```python
from build123d import *

# Parameters (mm, degrees)
PAD_DEPTH    = 10
SKETCH001_R  = 1.5
POCKET_DEPTH = 64.001


with BuildPart() as part:
    # Sketch → Pad (new body)
    with BuildSketch(Plane.XY):
        Polygon((80, 4), (-27.1, 4), (-27.1, -36), (-23.1, -36), (-23.1, 0), (0, 0), (0, -60), align=None)
        Polygon((2, 0), (2, -53.277501), (71.096876, 2), align=None, mode=Mode.SUBTRACT)
    extrude(amount=PAD_DEPTH)

    # Sketch001 (on Face5 of Pad) → Pocket (cut, through all)
    with BuildSketch(Plane(origin=(0, 4, 0), x_dir=(-1, 0, 0), z_dir=(0, 1, 0))):
        with Locations((-60, 5)):
            Circle(SKETCH001_R)
        with Locations((7.1, 5)):
            Circle(SKETCH001_R)
        with Locations((-26.45, 5)):
            Circle(SKETCH001_R)
    extrude(amount=-POCKET_DEPTH, mode=Mode.SUBTRACT)


solid = part.part
```
Part model, mm, in its own coordinate system. A direction names the side the tool comes from. Give positions to 0.01 mm unless a question says otherwise; leave off trailing zeros. Write each loop counter-clockwise with the first axis right and the second up, starting at its lowest first coordinate (ties: lowest second). Pieces come first, ordered by that corner, then holes. Notation, with made-up numbers: (28.25, 52.5) -> (60.25, 52.5) arc R15 ccw to (60.25, 70.5) -> close; hole circle Ø1 at (-15, 35.25). An arc over 180 degrees is marked (long way). Put each result on its own line as item: value. Start each with the question number.
Item 1: Cut at A-A (x = -7.1). List the corners of the cut face in (y, z).
Item 2: Wall check: L1, parallel to Z at x = 60, y = 2; L2, parallel to X at y = -10.25, z = 5; L3, parallel to X at y = -4, z = 4. Give the ranges that are in metal, low to high. Write a range as [from, to].
Item 3: Pin check, flat tips, straight feed: pin 1 Ø1.5 at (x, z) = (32.5, 3) entering from -Y; pin 2 Ø1.8 at (x, z) = (60, 5) entering from +Y; pin 3 Ø2 at (x, z) = (-25.5, 7) entering from -Y; pin 4 Ø3 at (y, z) = (-42, 6) entering from -X. Stop position of each tip, or through.
Item 4: Cut at B-B (z = 5). State how many separate pieces and enclosed holes the cut face has, then the cut area to 3 significant figures.
Item 5: Which spindle directions (+Z, -Z, +X, -X, +Y, -Y) get a long thin tool onto all of the face, cutting with end or side? Do faces 4 (the face through (36.1, -26, 4.9)), 5 (the face through (-25, -36, 5)), 6 (the face through (-12, 0, 5)). Say none if no direction does.
Item 6: Pull direction Z, two halves, no side cores. Call faces 1 (the face through (2, -26, 5)), 2 (the face through (18, 1, 10)), 3 (the face through (58.57, 2.83, 5.45)): pulls with the +Z half, pulls with the -Z half, needs draft (parallel to the pull), parting line crosses it, or undercut.
Item 7: Cut at C-C (y = -50.5). List the corners of the cut face in (x, z) (3 decimals).
Item 8: Cut at D-D (y = -17.5). List the corners of the cut face in (x, z) (3 decimals).
Answer list:
1. outline: (0, 0) -> (4, 0) -> (4, 3.5) -> (0, 3.5) -> close; (0, 6.5) -> (4, 6.5) -> (4, 10) -> (0, 10) -> close
2. L1: z = [0, 3.5], [6.5, 10]
2. L2: x = [-27.1, -23.1], [0, 2], [55.78, 58.5], [61.5, 62.19]
2. L3: x = [-27.1, -23.1], [0, 2], [63.6, 70]
3. pin 1: stops at y = -34.6
3. pin 2: passes through
3. pin 3: stops at y = -36
3. pin 4: stops at x = 0
4. separate pieces: 5
4. enclosed holes: 0
4. area: 912 mm2
5. face 4: +Z, -Z
5. face 5: +Z, -Z, -X, -Y
5. face 6: +Z, -Z, -Y
6. face 1: needs draft
6. face 2: pulls with the +Z half
6. face 3: undercut
7. outline: (0, 0) -> (2, 0) -> (2, 10) -> (0, 10) -> close; (5.472, 0) -> (11.875, 0) -> (11.875, 10) -> (5.472, 10) -> close
8. outline: (-27.1, 0) -> (-23.1, 0) -> (-23.1, 10) -> (-27.1, 10) -> close; (0, 0) -> (2, 0) -> (2, 10) -> (0, 10) -> close; (46.722, 0) -> (53.125, 0) -> (53.125, 10) -> (46.722, 10) -> close
